Geometry check sheet. Reference: the model listing, model coordinates, mm. Face numbers are marked on the shaded views. A direction names the side the tool comes from. Coordinates: 2 decimals unless noted, no trailing zeros. Loops run counter-clockwise (first coordinate to the right, second up) from the corner with the lowest first, then second, coordinate; pieces in that order, holes last.
from build123d import *

# Parameters (mm, degrees)
SKETCH004_W  = 545
SKETCH004_H  = 75
PAD004_DEPTH = 40
SKETCH005_W  = 40
SKETCH005_H  = 75
PAD005_DEPTH = 216
SKETCH006_W  = 72
SKETCH006_H  = 268
PAD006_DEPTH = 17
FILLET003_R  = 5
FILLET004_R  = 20


with BuildPart() as part:
    # Sketch004 (on Face1 of CopyPad003) → Pad004 (new body)
    with BuildSketch(Plane.XY.offset(415)):
        Rectangle(SKETCH004_W, SKETCH004_H)
    extrude(amount=PAD004_DEPTH)

    # Sketch005 (on Face6 of Pad004) → Pad005 (join)
    with BuildSketch(Plane.XY.offset(455)):
        with Locations((-252.5, 0)):
            Rectangle(SKETCH005_W, SKETCH005_H)
        with Locations((252.5, 0)):
            Rectangle(SKETCH005_W, SKETCH005_H)
    extrude(amount=PAD005_DEPTH)

    # Sketch006 (on Face5 of Pad005) → Pad006 (join)
    with BuildSketch(Plane.XY.offset(671)):
        with Locations((-252.5, 0)):
            Rectangle(SKETCH006_W, SKETCH006_H)
        with Locations((252.5, 0)):
            Rectangle(SKETCH006_W, SKETCH006_H)
    extrude(amount=PAD006_DEPTH)

    # Fillet003
    fillet003_edges = [part.edges().sort_by_distance(p)[0] for p in [
        (-288.5, 0, 688),
        (-216.5, 0, 688),
        (216.5, 0, 688),
        (288.5, 0, 688),
        (252.5, -134, 688),
        (252.5, 134, 688),
        (-252.5, 134, 688),
        (-252.5, -134, 688),
        (216.5, -134, 679.5),
        (288.5, -134, 679.5),
        (288.5, 134, 679.5),
        (216.5, 134, 679.5),
        (288.5, 0, 671),
        (252.5, 134, 671),
        (252.5, -134, 671),
        (216.5, 0, 671),
        (-288.5, 0, 671),
        (-252.5, -134, 671),
        (-288.5, -134, 679.5),
        (-216.5, -134, 679.5),
        (-216.5, 134, 679.5),
        (-216.5, 0, 671),
        (-252.5, 134, 671),
        (-288.5, 134, 679.5),
    ]]
    fillet(fillet003_edges, radius=FILLET003_R)

    # Fillet004
    fillet004_edges = [part.edges().sort_by_distance(p)[0] for p in [
        (-272.5, 0, 415),
        (-232.5, 0, 455),
        (232.5, 0, 455),
        (272.5, 0, 415),
        (272.5, -37.5, 543),
        (272.5, 37.5, 543),
        (-272.5, -37.5, 543),
        (-272.5, 37.5, 543),
    ]]
    fillet(fillet004_edges, radius=FILLET004_R)


solid = part.part
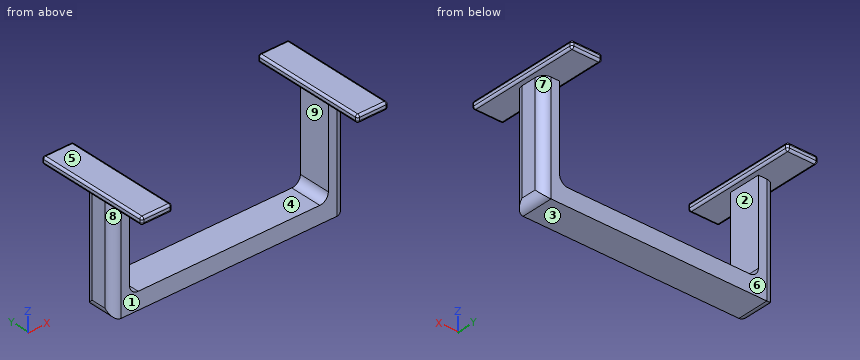
(1) Gauge pin test, flat ends, axial feed: pin 1 Ø10.5 at (y, z) = (2, 517.5) entering from +X; pin 2 Ø1.5 at (y, z) = (34, 631.5) entering from -X; pin 3 Ø10.5 at (y, z) = (3, 551.5) entering from -X. Record the tip position at first contact, or that the pin passes through.
Findings:
pin 1: stops at x = 272.5
pin 2: stops at x = -264.83
pin 3: stops at x = -272.5
(2) Sectioned sample at C-C on z = 447. Record the cut outline in (x, y), and give its area (3 significant figures).
Findings:
outline: (-272.5, -17.5) arc R20 ccw to (-252.5, -37.5) - (252.5, -37.5) arc R20 ccw to (272.5, -17.5) - (272.5, 17.5) arc R20 ccw to (252.5, 37.5) - (-252.5, 37.5) arc R20 ccw to (-272.5, 17.5) - close
area: 40,500 mm2
(3) Sectioned sample at B-B on z = 607.5. Record the cut outline in (x, y).
Findings:
outline: (-272.5, -17.5) arc R20 ccw to (-252.5, -37.5) - (-232.5, -37.5) - (-232.5, 37.5) - (-252.5, 37.5) arc R20 ccw to (-272.5, 17.5) - close; (232.5, -37.5) - (252.5, -37.5) arc R20 ccw to (272.5, -17.5) - (272.5, 17.5) arc R20 ccw to (252.5, 37.5) - (232.5, 37.5) - close
(4) Sectioned sample at A-A on y = 113.5. Record the cut outline in (x, z).
Findings:
outline: (-288.5, 676) arc R5 ccw to (-283.5, 671) - (-221.5, 671) arc R5 ccw to (-216.5, 676) - (-216.5, 683) arc R5 ccw to (-221.5, 688) - (-283.5, 688) arc R5 ccw to (-288.5, 683) - close; (216.5, 676) arc R5 ccw to (221.5, 671) - (283.5, 671) arc R5 ccw to (288.5, 676) - (288.5, 683) arc R5 ccw to (283.5, 688) - (221.5, 688) arc R5 ccw to (216.5, 683) - close
(5) Draft check along Z on the marked faces 1, 2, 3 and 4. Enter one of: +Z half, -Z half, draft (parallel to the pull), parting line (faces both ways), or undercut.
Findings:
face 1: draft
face 2: undercut
face 3: -Z half
face 4: +Z half
(6) Sectioned sample at D-D on x = -37. Record the cut outline in (y, z).
Findings:
outline: (-37.5, 415) - (37.5, 415) - (37.5, 455) - (-37.5, 455) - close
(7) Scan lines: L1, parallel to X at y = -17, z = 632; L2, parallel to Z at x = 50.5, y = 24; L3, parallel to Z at x = 226.5, y = -55. Record each from-to range of solid material in increasing order.
Findings:
L1: x = -272.5 to -232.5, 232.5 to 272.5
L2: z = 415 to 455
L3: z = 671 to 688
(8) Access from +Z, -Z, +X, -X, +Y, -Y to the whole of each face (thin tool, end or side, straight path). Record for the marked faces 5, 6, 7, 8 and 9.
Findings:
face 5: +Z, +X, -X, +Y, -Y
face 6: -Z, +X, -X, +Y
face 7: -Z, +X, +Y
face 8: -Z, -X, -Y
face 9: +Y, -Y
